Here's the drawing with two shaded views (mm, measured from the low corner). I have some questions. A direction names the side the tool comes from. Round coordinates to 2 decimals unless told otherwise and drop trailing zeros. Loops run counter-clockwise (first coordinate to the right, second up) from the corner with the lowest first, then second, coordinate; pieces in that order, holes last. Notation, with made-up numbers: M -38,38 L 12,38 A10 ccw 12,57 Z; hole C 56,-3.5 d5. An arc over 180 degrees is marked long. Answer as a JSON object with one key per item and string values.
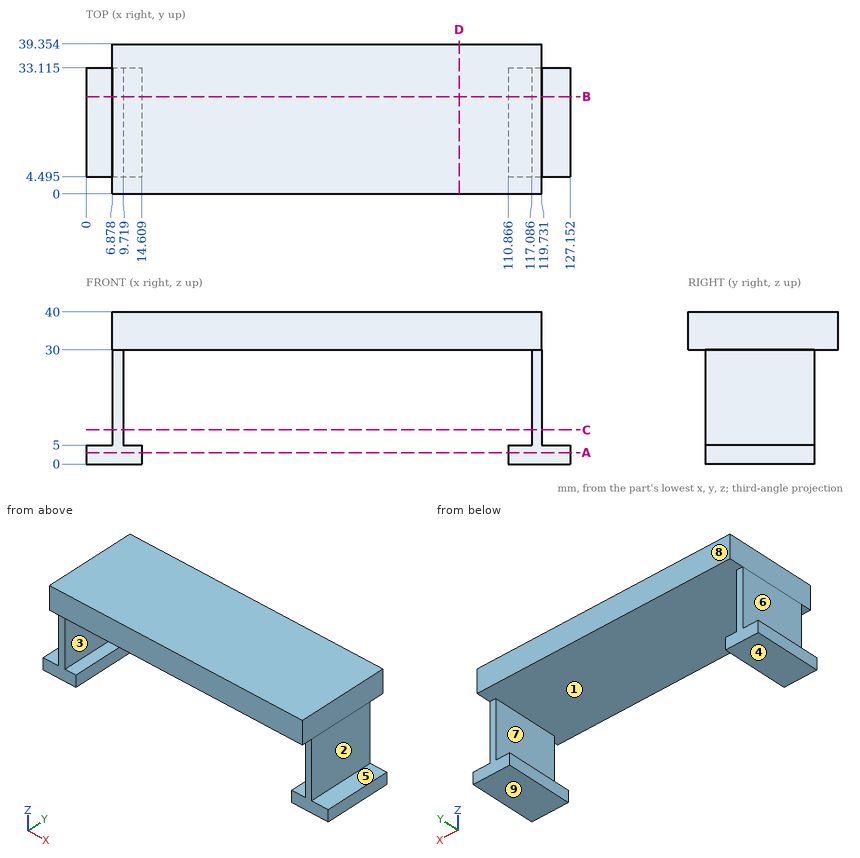
Item 1: For the marked faces 5, 6, 7, 8 and 9, which set-ups out of +Z, -Z, +X, -X, +Y, -Y let a thin tool reach every point of the face, with its end or its side?
Solution:
{"face 5": "+Z, +X, +Y, -Y", "face 6": "+Z, -X, +Y, -Y", "face 7": "+Y, -Y", "face 8": "+Z, -Z, +X, -X, +Y", "face 9": "-Z, +X, -X, +Y, -Y"}
Item 2: For P1, Ø7.5, axis at x = 2.5, y = 13, coming from the +Z side; P2, Ø13, axis at x = 117.5, z = 9, coming from the -Y side (1 decimal); P3, Ø11.5, axis at x = 7, z = 8, coming from the +Y side (1 decimal), each with a flat end and sliding along its axis, tell me the tip position at first contact or that it passes through.
Solution:
{"P1": "stops at z = 5", "P2": "stops at y = 4.5", "P3": "stops at y = 33.1"}
Item 3: We'd pull the mould along X, two halves only. Please class the marked faces 1, 2, 3 and 4: +X half, -X half, draft (parallel to the pull), parting line (faces both ways), or undercut.
Solution:
{"face 1": "undercut", "face 2": "+X half", "face 3": "undercut", "face 4": "draft"}
Item 4: I want a section at D-D on x = 98. List the corners of the cut face in (y, z) for me.
Solution:
{"outline": "M 0,30 L 39.35,30 L 39.35,40 L 0,40 Z"}
Item 5: If I drill on L1, parallel to X at y = 21.5, z = 4.5; L2, parallel to X at y = 27, z = 12; L3, parallel to Z at x = 112.5, y = 17.5, over which ranges is the centre line in solid material (lowest first)? Write a range as from..to.
Solution:
{"L1": "x = 0..14.61, 110.87..127.15", "L2": "x = 6.88..9.72, 117.09..119.73", "L3": "z = 0..5, 30..40"}
Item 6: I want a section at B-B on y = 25.5. List the corners of the cut face in (x, z) for me.
Solution:
{"outline": "M 0,0 L 14.61,0 L 14.61,5 L 9.72,5 L 9.72,30 L 117.09,30 L 117.09,5 L 110.87,5 L 110.87,0 L 127.15,0 L 127.15,5 L 119.73,5 L 119.73,40 L 6.88,40 L 6.88,5 L 0,5 Z"}
Item 7: I want a section at C-C on z = 9. List the corners of the cut face in (x, y) for me (1 decimal), plus the area to 3 significant figures.
Solution:
{"outline": "M 6.9,4.5 L 9.7,4.5 L 9.7,33.1 L 6.9,33.1 Z; M 117.1,4.5 L 119.7,4.5 L 119.7,33.1 L 117.1,33.1 Z", "area": "157 mm2"}
Item 8: I want a section at A-A on z = 3. List the corners of the cut face in (x, y) for me (1 decimal), plus the area to 3 significant figures.
Solution:
{"outline": "M 0,4.5 L 14.6,4.5 L 14.6,33.1 L 0,33.1 Z; M 110.9,4.5 L 127.2,4.5 L 127.2,33.1 L 110.9,33.1 Z", "area": "884 mm2"}
